Work out the finished part from the listing and answer in its coordinate system (mm). A direction names the side the tool comes from. Coordinates: 2 decimals unless noted, no trailing zeros. Order: outer loops, then holes, each group sorted by start corner. A loop starts at its lowest first (then second) coordinate and runs counter-clockwise, first axis right, second up. Notation, with made-up numbers: M -2.75,-3.75 L 23.25,-3.75 A33 cw 23.25,29.25 Z; hole C 3.25,52 d1. An arc over 180 degrees is marked long. Use a Markdown table: item, result.
from build123d import *

# Parameters (mm, degrees)
SKETCH1_R           = 1.9
BOSS_EXTRUDE1_DEPTH = 4.5
FILLET1_R           = 7


with BuildPart() as part:
    # Sketch1 → Boss-Extrude1 (new body)
    with BuildSketch(Plane(origin=(0, 0, 0), x_dir=(1, 0, 0), z_dir=(0, 1, 0))):
        Polygon((0, 0), (17.587865182, 0), (23.5, 2.533671894), (29.412134818, 0), (47, 0), (47, 7.6), (27.25, 7.6), (27.25, 28.25), (25, 28.25), (25, 22.25), (22, 22.25), (22, 28.25), (19.75, 28.25), (19.75, 7.6), (0, 7.6), align=None)
        with Locations(Location((4, 3.6, 0), (0, 0, 270))):
            Circle(SKETCH1_R, mode=Mode.SUBTRACT)
        with Locations(Location((14, 3.6, 0), (0, 0, 270))):
            Circle(SKETCH1_R, mode=Mode.SUBTRACT)
        with Locations(Location((33, 3.6, 0), (0, 0, 270))):
            Circle(SKETCH1_R, mode=Mode.SUBTRACT)
        with Locations(Location((43, 3.6, 0), (0, 0, 270))):
            Circle(SKETCH1_R, mode=Mode.SUBTRACT)
    boss_extrude1 = extrude(amount=BOSS_EXTRUDE1_DEPTH)

    # Mirror1: Boss-Extrude1 across plane
    add(boss_extrude1.mirror(Plane(origin=(19.75, 4.5, -28.25), x_dir=(1, 0, 0), z_dir=(0, 0, 1))))

    # Fillet1
    fillet1_edges = [part.edges().sort_by_distance(p)[0] for p in [
        (29.412134818, 2.25, 0),
        (23.5, 2.25, -2.533671894),
        (17.587865182, 2.25, 0),
        (29.412134818, 2.25, -56.5),
        (23.5, 2.25, -53.966328106),
        (17.587865182, 2.25, -56.5),
    ]]
    fillet(fillet1_edges, radius=FILLET1_R)


solid = part.part
1. Section A-A on x = 10.5 is taken. Determine the outline of the cut face in (y, z).
Answers below:
| item | result |
|---|---|
| outline | M 0,-56.5 L 4.5,-56.5 L 4.5,-48.9 L 0,-48.9 Z; M 0,-7.6 L 4.5,-7.6 L 4.5,0 L 0,0 Z |
2. Section D-D on z = -25 is taken. Determine the outline of the cut face in (x, y), then the cut area to 4 significant figures.
Answers below:
| item | result |
|---|---|
| outline | M 19.75,0 L 22,0 L 22,4.5 L 19.75,4.5 Z; M 25,0 L 27.25,0 L 27.25,4.5 L 25,4.5 Z |
| area | 20.25 mm² |
3. For a pull along X with two mould halves and no side action, classify faces 1 (the face through (10, 2, -7.6)), 2 (the face through (19.75, 2, -28)), 3 (the face through (23.46, 2.282, -1.918)) as +X half, -X half, draft (parallel to the pull), parting line (faces both ways), or undercut.
Answers below:
| item | result |
|---|---|
| face 1 | draft |
| face 2 | -X half |
| face 3 | undercut |
4. Section B-B on z = -3.6 is taken. Determine the outline of the cut face in (x, y).
Answers below:
| item | result |
|---|---|
| outline | M 0,0 L 2.1,0 L 2.1,4.5 L 0,4.5 Z; M 5.9,0 L 12.1,0 L 12.1,4.5 L 5.9,4.5 Z; M 15.9,0 L 31.1,0 L 31.1,4.5 L 15.9,4.5 Z; M 34.9,0 L 41.1,0 L 41.1,4.5 L 34.9,4.5 Z; M 44.9,0 L 47,0 L 47,4.5 L 44.9,4.5 Z |
5. For faces 4 (the face through (24, 2, -34.25)), 5 (the face through (17.54, 2.28, -56.36)), 6 (the face through (17.54, 2.28, -0.14)), 7 (the face through (37, 2, -7.6)), determine the directions among +Z, -Z, +X, -X, +Y, -Y from which every point of the face is accessible in a straight line to the end or side of a thin tool.
Answers below:
| item | result |
|---|---|
| face 4 | +Y, -Y |
| face 5 | -Z, +Y, -Y |
| face 6 | +Z, +Y, -Y |
| face 7 | +X, +Y, -Y |
6. A flat-ended cylindrical pin translates along its axis: P1, Ø2.5, axis at x = 24, y = 2, coming from the +Z side. Find the tip coordinate at first contact, or state that the pin passes through.
Answers below:
| item | result |
|---|---|
| P1 | z = -1.7 |
7. Find the intervals of material crossed by probe 1 along X at (y, z) = (1.8, -3.6); probe 2 along Z at (x, y) = (7.5, 2.65); probe 3 along X at (y, z) = (2.15, -24.5), in increasing order.
Answers below:
| item | result |
|---|---|
| probe 1 | 0 to 2.1, 5.9 to 12.1, 15.9 to 31.1, 34.9 to 41.1, 44.9 to 47 |
| probe 2 | -56.5 to -48.9, -7.6 to 0 |
| probe 3 | 19.75 to 22, 25 to 27.25 |
8. Section C-C on x = 33 is taken. Determine the outline of the cut face in (y, z).
Answers below:
| item | result |
|---|---|
| outline | M 0,-56.5 L 4.5,-56.5 L 4.5,-54.8 L 0,-54.8 Z; M 0,-51 L 4.5,-51 L 4.5,-48.9 L 0,-48.9 Z; M 0,-7.6 L 4.5,-7.6 L 4.5,-5.5 L 0,-5.5 Z; M 0,-1.7 L 4.5,-1.7 L 4.5,0 L 0,0 Z |
